Verification items for the finished model (mm, model axes). A direction names the side the tool comes from. Round coordinates to 2 decimals unless told otherwise and drop trailing zeros. Write each loop counter-clockwise with the first axis right and the second up, starting at its lowest first coordinate (ties: lowest second). Pieces come first, ordered by that corner, then holes. Notation, with made-up numbers: M 52.25,50 L 100.25,50 A13 cw 100.25,60 Z; hole C 50.5,-21.75 d7. An arc over 180 degrees is marked long. One line per item, written item: value. Start each with the question number.
Item 1: Thickness scan on probe 1 along X at (y, z) = (-11, 0.6); probe 2 along X at (y, z) = (9.5, 2.3); probe 3 along Y at (x, z) = (26, 2.5). Record the ranges inside material, lowest first. Write a range as from..to.
Item 2: Gauge pin test, flat end, axial feed: pin 1 (12.5 mm diameter, centred on x = -33.5, y = 13, fed in from -Z). Record the tip position at first contact, or that the pin passes through.
Item 3: Tool access check on faces 4 (the face through (-27, 28.703, 1)), 5 (the face through (-20.44, 19.32, 2.51)). Record the directions out of +Z, -Z, +X, -X, +Y, -Y that give a thin tool (end or side, any length) a straight path to the whole face; none if there is none.
Item 4: Section check C-C, the plane z = 1.5. Record the cut outline in (x, y).
Item 5: Draft check along Y on faces 1 (the face through (-5, 9, 3)), 2 (the face through (-5, -16.297, 1)), 3 (the face through (-48.156, 8, 1)). Enter one of: +Y half, -Y half, draft (parallel to the pull), parting line (faces both ways), or undercut.
Item 6: Section check D-D, the plane y = 14. Record the cut outline in (x, z).
Item 7: Section check A-A, the plane y = 27.5. Record the cut outline in (x, z), then the cut area to 3 significant figures.
Item 8: Section check B-B, the plane x = 7. Record the cut outline in (y, z), then the cut area to 3 significant figures.
from build123d import *

# Parameters (mm, degrees)
SKETCH_W        = 92.866455
SKETCH_H        = 49.076486
PAD_DEPTH       = 3
SKETCH001_R     = 1.87588
SKETCH001_R_2   = 1.936405
SKETCH001_R_3   = 12.5
SKETCH001_R_4   = 5.95
SKETCH001_R_5   = 5
SKETCH001_R_6   = 10.4
SKETCH001_R_7   = 10.9
SKETCH001_R_8   = 2.6
POCKET_DEPTH    = 5
SKETCH002_W     = 42
SKETCH002_H     = 42
POCKET001_DEPTH = 2


with BuildPart() as part:
    # Sketch → Pad (new body)
    with BuildSketch(Plane.XY):
        with Locations((-4.722953, 8.240901)):
            Rectangle(SKETCH_W, SKETCH_H)
    extrude(amount=PAD_DEPTH)

    # Sketch001 (on Face6 of Pad) → Pocket (cut)
    with BuildSketch(Plane.XY.offset(3)):
        with Locations((-42.156181, 23.779144)):
            Circle(SKETCH001_R)
        with Locations((-12.156181, 23.779144)):
            Circle(SKETCH001_R)
        with Locations((-12.156181, -6.220856)):
            Circle(SKETCH001_R_2)
        with Locations((-42.156181, -6.220856)):
            Circle(SKETCH001_R_2)
        with Locations((-27.156181, 8.779144)):
            Circle(SKETCH001_R_3)
        with Locations((4.704166, 24.273006)):
            Circle(SKETCH001_R_4)
        with Locations((28.842405, 2.41649)):
            Circle(SKETCH001_R_5)
        with Locations((27.041033, 20.069828)):
            Circle(SKETCH001_R_6)
        with Locations((7.826513, 4.698213)):
            Circle(SKETCH001_R_7)
        with Locations((21.396776, -8.031404)):
            Circle(SKETCH001_R_8)
    extrude(amount=-POCKET_DEPTH, mode=Mode.SUBTRACT)

    # Sketch002 (on Face4 of Pocket) → Pocket001 (cut)
    with BuildSketch(Plane(origin=(0, 0, 0), x_dir=(1, 0, 0), z_dir=(0, 0, -1))):
        with Locations((-27.156181, -7.702658)):
            Rectangle(SKETCH002_W, SKETCH002_H)
    extrude(amount=-POCKET001_DEPTH, mode=Mode.SUBTRACT)


solid = part.part
Response values:
1. probe 1: x = -51.16..-48.16, -6.16..41.71
1. probe 2: x = -51.16..-39.64, -14.68..-1.96, 17.61..41.71
1. probe 3: y = -16.3..-1.7, 6.53..9.72, 30.42..32.78
2. pin 1: stops at z = 2
3. face 4: -Z
3. face 5: +Z, -Z
4. outline: M -51.16,-16.3 L 41.71,-16.3 L 41.71,32.78 L -51.16,32.78 Z; hole M -48.16,-13.3 L -6.16,-13.3 L -6.16,28.7 L -48.16,28.7 Z; hole C 7.83,4.7 d21.8; hole C 4.7,24.27 d11.9; hole C 27.04,20.07 d20.8; hole C 21.4,-8.03 d5.2; hole C 28.84,2.42 d10
5. face 1: draft
5. face 2: -Y half
5. face 3: undercut
6. outline: M -51.16,0 L -48.16,0 L -48.16,2 L -38.51,2 L -38.51,3 L -51.16,3 Z; M -15.8,2 L -6.16,2 L -6.16,0 L 2.14,0 L 2.14,3 L -15.8,3 Z; M 13.51,0 L 18.6,0 L 18.6,3 L 13.51,3 Z; M 35.49,0 L 41.71,0 L 41.71,3 L 35.49,3 Z
7. outline: M -51.16,0 L -48.16,0 L -48.16,2 L -6.16,2 L -6.16,0 L -0.29,0 L -0.29,3 L -51.16,3 Z; M 9.7,0 L 19.76,0 L 19.76,3 L 9.7,3 Z; M 34.32,0 L 41.71,0 L 41.71,3 L 34.32,3 Z
7. area: 121 mm2
8. outline: M -16.3,0 L -6.17,0 L -6.17,3 L -16.3,3 Z; M 15.57,0 L 18.78,0 L 18.78,3 L 15.57,3 Z; M 29.76,0 L 32.78,0 L 32.78,3 L 29.76,3 Z
8. area: 49.1 mm2
